Geometry: final body of the model. Coordinates: model frame, mm. A direction names the side the tool comes from. Give positions to 0.01 mm unless a question says otherwise; leave off trailing zeros. Loops run counter-clockwise (first coordinate to the right, second up) from the corner with the lowest first, then second, coordinate; pieces in that order, holes last. Notation, with made-up numbers: (23, 18.25) -> (70, 18.25) arc R16 ccw to (70, 32.25) -> close; hole circle Ø6 at (29.5, 78). An arc over 180 degrees is marked (long way). Answer in a Markdown table with one row per item. Add a question column.
1) Access query for faces 1 (the flat face through (4.5, -2, 3)), 2 (the cylindrical face through (-0.54, 0.56, 8.22)). Directions: +Z, -Z, +X, -X, +Y, -Y. A direction counts if a zero-diameter tool reaches every point of the face in a straight line with its end or side. Return the directions, or none.
2) First-contact query: P1, Ø4, axis at x = 2.5, z = 2, coming from the +Y side; P2, Ø1.5, axis at y = 0.5, z = 7.5, coming from the +X side; P3, Ø1.5, axis at y = 1.5, z = 8.5, coming from the +X side. Flat tips, straight axial feed; report the tip coordinate or a pass-through.
3) Section query B-B (x = -1.75). Return the cut outline in (y, z), plus the area to 3 significant figures.
4) Section query A-A (y = 5). Return the cut outline in (x, z).
5) Line query: line 1 (Z direction, x = 0, y = 6.5); line 2 (X direction, y = 5, z = 8.5); line 3 (Y direction, x = 0.75, z = 2.75). Output: solid intervals per line, ascending. Write a range as from..to.
6) Section query D-D (z = 9.5). Return the cut outline in (x, y), plus the area to 3 significant figures.
```python
from build123d import *

# Parameters (mm, degrees)
F0_W     = 9
F0_H     = 15
F1_DEPTH = 6
F2_R     = 2.5
F3_DEPTH = 4.5
F4_R     = 4.49999


# Not quite as in the source:
# - a fillet or chamfer is up to 0.001 mm smaller than in the source, because OpenCascade refuses the exact size


with BuildPart() as f1:
    # F0 (on Top) → F1 (new body)
    with BuildSketch(Plane.XY):
        Rectangle(F0_W, F0_H)
    extrude(amount=F1_DEPTH)

    # F2 (on face) → F3 (join)
    with BuildSketch(Plane.XY.offset(6)):
        with Locations((0, 3)):
            Circle(F2_R)
    extrude(amount=F3_DEPTH)

    # F4 (radius 4.5 in the source; OpenCascade refuses exactly that, so slightly less here)
    f4_edges = [f1.edges().sort_by_distance(p)[0] for p in [
        (-4.5, 7.5, 3),
        (4.5, 7.5, 3),
    ]]
    fillet(f4_edges, radius=F4_R)


solid = f1.part
```
Evaluation:
| question | item | result |
|---|---|---|
| 1 | face 1 | +Z, -Z, +X, +Y, -Y |
| 1 | face 2 | +Z |
| 2 | P1 | y = 7.47 |
| 2 | P2 | x = 1.79 |
| 2 | P3 | x = 2.38 |
| 3 | outline | (-7.5, 0) -> (7.15, 0) -> (7.15, 6) -> (4.79, 6) -> (4.79, 10.5) -> (1.21, 10.5) -> (1.21, 6) -> (-7.5, 6) -> close |
| 3 | area | 104 mm² |
| 4 | outline | (-4.03, 0) -> (4.03, 0) -> (4.03, 6) -> (1.5, 6) -> (1.5, 10.5) -> (-1.5, 10.5) -> (-1.5, 6) -> (-4.03, 6) -> close |
| 5 | line 1 | 0..6 |
| 5 | line 2 | -1.5..1.5 |
| 5 | line 3 | -7.5..7.44 |
| 6 | outline | circle Ø5 at (0, 3) |
| 6 | area | 19.6 mm² |
